For this review, use the dimensioned drawing (mm, ordinates from the lowest corner) and the shaded views. Give positions to 0.01 mm unless a question says otherwise; leave off trailing zeros. Order: outer loops, then holes, each group sorted by start corner. A loop starts at its lowest first (then second) coordinate and runs counter-clockwise, first axis right, second up. Notation, with made-up numbers: (26.5, -19.5) - (48.5, -19.5) arc R11 cw to (48.5, -15.5) - close; hole circle Ø10 at (74, -28). An arc over 180 degrees is marked (long way). One line per item, written item: value.
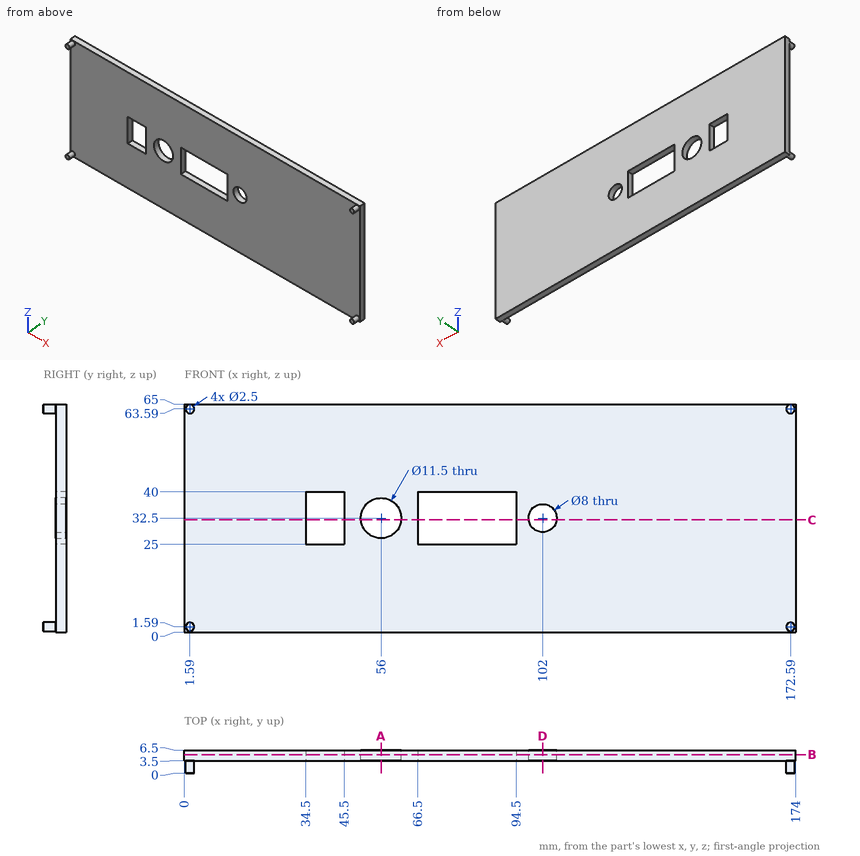
(1) Take a section at B-B (y = 5.25). Write out the cut boundary in (x, z).
Answers below:
outline: (0, 0) - (174, 0) - (174, 65) - (0, 65) - close; hole (34.5, 25) - (45.5, 25) - (45.5, 40) - (34.5, 40) - close; hole circle Ø11.5 at (56, 32.5); hole (66.5, 25) - (94.5, 25) - (94.5, 40) - (66.5, 40) - close; hole circle Ø8 at (102, 32.5)
(2) For P1, Ø0.9, axis at x = 41, y = 5.5, coming from the -Z side; P2, Ø8, axis at x = 87, z = 46.5, coming from the -Y side, all flat-tipped, find the tip position at first contact; note any pin that passes through.
Answers below:
P1: stops at z = 0
P2: stops at y = 3.5
(3) Wall thickness on line 1 (X direction, y = 4.2, z = 32.5); line 2 (X direction, y = 4.75, z = 38.5); line 3 (Y direction, x = 167, z = 47): over which ranges is each line inside the solid? List them lowest first. Write a range as from..to.
Answers below:
line 1: x = 0..34.5, 45.5..50.25, 61.75..66.5, 94.5..98, 106..174
line 2: x = 0..34.5, 45.5..66.5, 94.5..174
line 3: y = 3.5..6.5
(4) Take a section at D-D (x = 102). Write out the cut boundary in (y, z), then the cut area to 3 significant figures.
Answers below:
outline: (3.5, 0) - (6.5, 0) - (6.5, 28.5) - (3.5, 28.5) - close; (3.5, 36.5) - (6.5, 36.5) - (6.5, 65) - (3.5, 65) - close
area: 171 mm^2
(5) Take a section at C-C (z = 32). Write out the cut boundary in (x, y).
Answers below:
outline: (0, 3.5) - (34.5, 3.5) - (34.5, 6.5) - (0, 6.5) - close; (45.5, 3.5) - (50.27, 3.5) - (50.27, 6.5) - (45.5, 6.5) - close; (61.73, 3.5) - (66.5, 3.5) - (66.5, 6.5) - (61.73, 6.5) - close; (94.5, 3.5) - (98.03, 3.5) - (98.03, 6.5) - (94.5, 6.5) - close; (105.97, 3.5) - (174, 3.5) - (174, 6.5) - (105.97, 6.5) - close
(6) Take a section at A-A (x = 56). Write out the cut boundary in (y, z).
Answers below:
outline: (3.5, 0) - (6.5, 0) - (6.5, 26.75) - (3.5, 26.75) - close; (3.5, 38.25) - (6.5, 38.25) - (6.5, 65) - (3.5, 65) - close
